For this review, take the finished solid that the model builds, in its own axes (mm). Round coordinates to 2 decimals unless told otherwise and drop trailing zeros. Order: outer loops, then holes, each group sorted by start corner. A loop starts at its lowest first (then second) coordinate and runs counter-clockwise, first axis right, second up. Notation, with made-up numbers: (70, 2) - (75, 2) arc R20 cw to (75, 18) - close; hole circle Ø10 at (-23.5, -3.5). An arc over 180 degrees is marked (long way). Write each question's results on one line, items separated by ' | '. Start each with the question number.
(1) Take a section at B-B, the plane x = -1.27. Give the boundary of the cut face in (y, z), plus the area to 3 significant figures.
(2) Take a section at C-C, the plane x = -3.81. Give the boundary of the cut face in (y, z).
(3) For L1, parallel to Y at x = 1.25, z = -0.9; L2, parallel to Y at x = -3.81, z = -0.5; L3, parallel to X at y = -5.5, z = -0.25, list the stretches that pass through material, from the lowest coordinate up. Write a range as from..to.
(4) Take a section at A-A, the plane y = 5.5. Give the boundary of the cut face in (x, z), plus the area to 3 significant figures.
(5) Take a section at D-D, the plane x = -9. Give the boundary of the cut face in (y, z), plus the area to 3 significant figures.
(6) Insertion check: pin 1 Ø1.5 at (x, y) = (-7.5, 11) entering from +Z. The pin has a flat end and moves straight along its axis. Give the tip position at first contact, or say it passes through.
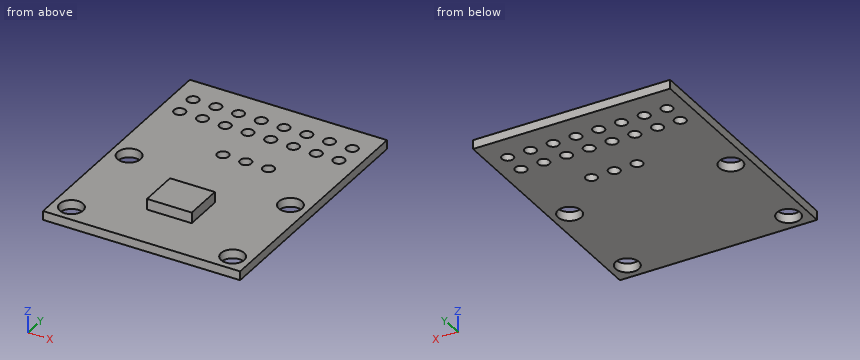
Autodesk Inventor part; units mm, degrees
ref_plane "YZ Plane" through (0, 0, 0) normal (1, 0, 0) x (0, 1, 0)
ref_plane "XZ Plane" through (0, 0, 0) normal (0, 1, 0) x (-1, 0, 0)
ref_plane "XY Plane" through (0, 0, 0) normal (0, 0, 1) x (1, 0, 0)
sketch "スケッチ1" plane through (0, 0, 0) normal (0, 0, 1) x (1, 0, 0)
  line L0 (-11, -7.5) -> (11, -7.5)
  line L1 (11, -7.5) -> (11, 20.5)
  line L2 (11, 20.5) -> (-11, 20.5)
  line L3 (-11, 20.5) -> (-11, -7.5)
  line L4 (-11, -7.5) -> (11, 20.5) construction
  line L5 (11, -7.5) -> (-11, 20.5) construction
  line L6 (-9, -5.5) -> (9, -5.5) construction
  line L7 (9, -5.5) -> (9, 5.5) construction
  line L8 (9, 5.5) -> (-9, 5.5) construction
  line L9 (-9, 5.5) -> (-9, -5.5) construction
  line L10 (-9, -5.5) -> (9, 5.5) construction
  line L11 (9, -5.5) -> (-9, 5.5) construction
  point P0 (0, 0)
  point P1 (0, 6.5)
  point P2 (0, 6.5)
  point P3 (0, 0)
  point P4 (0, 0)
  point P5 (0, 0)
  dimension "d0" = 22
  dimension "d1" = 28
  dimension "d2" = 18
  dimension "d3" = 11
  dimension "d4" = 2
extrude "押し出し1" add sketch "スケッチ1" against normal blind 1
sketch "スケッチ2" plane through (0, 0, 0) normal (0, 0, 1) x (1, 0, 0)
  line L0 (-9, -5.5) -> (9, -5.5)
  line L1 (9, -5.5) -> (9, 5.5)
  line L2 (9, 5.5) -> (-9, 5.5)
  line L3 (-9, 5.5) -> (-9, -5.5)
  line L4 (-9, -5.5) -> (9, 5.5) construction
  line L5 (9, -5.5) -> (-9, 5.5) construction
  point P0 (0, 0)
  dimension "d7" = 11
  dimension "d8" = 18
hole "穴1" at (-9, 5.5, 0) at (-9, -5.5, 0) at (9, 5.5, 0) at (9, -5.5, 0) direction (0, 0, -1) diameter 2.6 end through all
sketch "スケッチ3" plane through (0, 0, 0) normal (0, 0, 1) x (1, 0, 0)
  line L0 (-2.5, -2.2) -> (2.5, -2.2)
  line L1 (2.5, -2.2) -> (2.5, 2.2)
  line L2 (2.5, 2.2) -> (-2.5, 2.2)
  line L3 (-2.5, 2.2) -> (-2.5, -2.2)
  line L4 (-2.5, -2.2) -> (2.5, 2.2) construction
  line L5 (2.5, -2.2) -> (-2.5, 2.2) construction
  point P0 (0, 0)
  dimension "d16" = 4.4
  dimension "d17" = 5
extrude "押し出し2" add sketch "スケッチ3" along normal blind 1.2
sketch "スケッチ4" plane through (0, 0, 0) normal (0, 0, 1) x (1, 0, 0)
  line L0 (-11, 20.5) -> (-11, -7.5)
  line L1 (-11, 20.5) -> (11.0137, 20.4892) construction
  line L2 (11.0137, 20.4892) -> (11, -7.5) construction
  line L3 (11, -7.5) -> (-11.0137, -7.4892) construction
  line L4 (-11.0137, -7.4892) -> (-11, 20.5) construction
  line L5 (11, -7.5) -> (11, 20.5)
  line L6 (-11, -7.5) -> (11, -7.5)
  circle A0 centre (-1.27, 17.4952) radius 0.635
  circle A1 centre (1.27, 17.494) radius 0.635
  circle A2 centre (-1.27, 14.9552) radius 0.635
  circle A3 centre (1.27, 14.954) radius 0.635
  circle A4 centre (-3.81, 14.9565) radius 0.635
  circle A5 centre (-3.81, 17.4965) radius 0.635
  circle A6 centre (-6.35, 14.9577) radius 0.635
  circle A7 centre (-6.35, 17.4977) radius 0.635
  circle A8 centre (-8.89, 14.959) radius 0.635
  circle A9 centre (-8.89, 17.499) radius 0.635
  circle A10 centre (3.81, 17.4928) radius 0.635
  circle A11 centre (3.81, 14.9528) radius 0.635
  circle A12 centre (6.35, 17.4915) radius 0.635
  circle A13 centre (6.35, 14.9515) radius 0.635
  circle A14 centre (8.89, 17.4903) radius 0.635
  circle A15 centre (8.89, 14.9503) radius 0.635
  circle A16 centre (-1.27, 10.1952) radius 0.635
  circle A17 centre (1.27, 10.194) radius 0.635
  circle A18 centre (3.81, 10.1928) radius 0.635
  point P0 (0, 0)
  dimension "d25" = 3
  dimension "d30" = 2.54
  dimension "d32" = 1.27
  dimension "d37" = 1.27
  dimension "d38" = 1.27
  dimension "d39" = 3
  dimension "d41" = 2.54
  dimension "d43" = 2.54
  dimension "d45" = 1.27
  dimension "d46" = 1.27
  dimension "d53" = 2.54
  dimension "d63" = 2.54
  dimension "d71" = 1.27
  dimension "d73" = 10.3
  dimension "d78" = 2.54
extrude "押し出し3" cut sketch "スケッチ4" against normal through all
equation "\"d45\" = d37"
equation "\"d46\" = d45"
equation "\"d71\" = d45"
properties part number "AS5047P-TS_EK_AB" material "ABS プラスチック"
Results below:
1) outline: (-7.5, -1) - (9.56, -1) - (9.56, 0) - (2.2, 0) - (2.2, 1.2) - (-2.2, 1.2) - (-2.2, 0) - (-7.5, 0) - close; (10.83, -1) - (14.32, -1) - (14.32, 0) - (10.83, 0) - close; (15.59, -1) - (16.86, -1) - (16.86, 0) - (15.59, 0) - close; (18.13, -1) - (20.5, -1) - (20.5, 0) - (18.13, 0) - close | area: 29.5 mm^2
2) outline: (-7.5, -1) - (14.32, -1) - (14.32, 0) - (-7.5, 0) - close; (15.59, -1) - (16.86, -1) - (16.86, 0) - (15.59, 0) - close; (18.13, -1) - (20.5, -1) - (20.5, 0) - (18.13, 0) - close
3) L1: y = -7.5..9.56, 10.83..14.32, 15.59..16.86, 18.13..20.5 | L2: y = -7.5..14.32, 15.59..16.86, 18.13..20.5 | L3: x = -11..-10.3, -7.7..7.7, 10.3..11
4) outline: (-11, -1) - (-10.3, -1) - (-10.3, 0) - (-11, 0) - close; (-7.7, -1) - (7.7, -1) - (7.7, 0) - (-7.7, 0) - close; (10.3, -1) - (11, -1) - (11, 0) - (10.3, 0) - close | area: 16.8 mm^2
5) outline: (-7.5, -1) - (-6.8, -1) - (-6.8, 0) - (-7.5, 0) - close; (-4.2, -1) - (4.2, -1) - (4.2, 0) - (-4.2, 0) - close; (6.8, -1) - (14.33, -1) - (14.33, 0) - (6.8, 0) - close; (15.58, -1) - (16.87, -1) - (16.87, 0) - (15.58, 0) - close; (18.12, -1) - (20.5, -1) - (20.5, 0) - (18.12, 0) - close | area: 20.3 mm^2
6) pin 1: stops at z = 0
